```python
from build123d import *

# Parameters (mm, degrees)
SKETCH_R             = 10.3
PAD_DEPTH            = 2.9
SKETCH001_R          = 7.4
PAD001_DEPTH         = 19
SKETCH002_W          = 13.2
SKETCH002_H          = 4.5
POCKET_DEPTH         = 20
SKETCH003_W          = 8
SKETCH003_H          = 4.5
POCKET001_DEPTH      = 1.901
POCKET002_DEPTH      = 6
SKETCH005_R          = 1.5
POCKET003_DEPTH      = 15
POCKET004_DEPTH      = 20
POCKET004_DEPTH_BACK = -20
SKETCH007_W          = 2.3
SKETCH007_H          = 1.5
POCKET005_DEPTH      = 10.301


with BuildPart() as part:
    # Sketch → Pad (new body)
    with BuildSketch(Plane.XY):
        Circle(SKETCH_R)
    extrude(amount=PAD_DEPTH)

    # Sketch001 (on Face3 of Pad) → Pad001 (join)
    with BuildSketch(Plane.XY.offset(2.9)):
        Circle(SKETCH001_R)
    extrude(amount=PAD001_DEPTH)

    # Sketch002 (on Face5 of Pad001) → Pocket (cut)
    with BuildSketch(Plane.XY.offset(21.9)):
        Rectangle(SKETCH002_W, SKETCH002_H)
    extrude(amount=-POCKET_DEPTH, mode=Mode.SUBTRACT)

    # Sketch003 (on Face10 of Pocket) → Pocket001 (cut, through all)
    with BuildSketch(Plane.XY.offset(1.9)):
        Rectangle(SKETCH003_W, SKETCH003_H)
    extrude(amount=-POCKET001_DEPTH, mode=Mode.SUBTRACT)

    # Sketch004 (on Face9 of Pocket001) → Pocket002 (cut)
    with BuildSketch(Plane.XY.offset(21.9)):
        with BuildLine():
            ThreePointArc((-6, 0), (0, -6), (6, 0))
            Line((-6, 0), (6, 0))
        make_face()
    extrude(amount=-POCKET002_DEPTH, mode=Mode.SUBTRACT)

    # Sketch005 (on Face13 of Pocket002) → Pocket003 (cut)
    with BuildSketch(Plane.XY.offset(15.9)):
        with Locations((0, -4)):
            Circle(SKETCH005_R)
    extrude(amount=-POCKET003_DEPTH, mode=Mode.SUBTRACT)

    # Sketch006 → Pocket004 (cut, two sides)
    with BuildSketch(Plane.XZ) as pocket004_sk:
        with BuildLine():
            ThreePointArc((-2.25, 19.25), (-4, 17.5), (-2.25, 15.75))
            Line((-2.25, 15.75), (2.25, 15.75))
            ThreePointArc((2.25, 15.75), (4, 17.5), (2.25, 19.25))
            Line((-2.25, 19.25), (2.25, 19.25))
        make_face()
    extrude(amount=-POCKET004_DEPTH, mode=Mode.SUBTRACT)
    extrude(pocket004_sk.sketch, amount=-POCKET004_DEPTH_BACK, mode=Mode.SUBTRACT)

    # Sketch007 → Pocket005 (cut, through all)
    with BuildSketch(Plane.XZ):
        with Locations((0, 20)):
            Rectangle(SKETCH007_W, SKETCH007_H)
    extrude(amount=-POCKET005_DEPTH, mode=Mode.SUBTRACT)


solid = part.part
```
For this review, take the finished solid that the model builds, in its own axes (mm). A direction names the side the tool comes from. Coordinates: 2 decimals unless noted, no trailing zeros. Write each loop counter-clockwise with the first axis right and the second up, starting at its lowest first coordinate (ties: lowest second). Pieces come first, ordered by that corner, then holes. Notation, with made-up numbers: (8.25, 52) - (12.25, 52) arc R29 cw to (12.25, 89) - close; hole circle Ø1 at (35, 3.5). An arc over 180 degrees is marked (long way). Answer in a Markdown table with one row per item. Add a question column.
Q1. For probe 1 along Y at (x, z) = (0, 7); probe 2 along Z at (x, y) = (-1.25, -9.5); probe 3 along Z at (x, y) = (-0.75, -5.25), list the stretches that pass through material, from the lowest coordinate up.
Q2. Tool access review of faces 1 (the cylindrical face through (-4, 4.6, 17.5)), 2 (the flat face through (-4, 0, 1)), 3 (the flat face through (-6.6, 0, 12)): name each direction out of +Z, -Z, +X, -X, +Y, -Y from which nothing blocks a thin tool from reaching the whole face with its end or side.
Q3. We need section D-D, the plane x = -6. State the section outline as (y, z) points.
Q4. We need section B-B, the plane y = 0. State the section outline as (x, z) points, and give its area (3 significant figures).
Q5. We need section A-A, the plane x = 0. State the section outline as (y, z) points.
Q6. For P1, Ø3.5, axis at y = -1, z = 16.5, coming from the -X side; P2, Ø10, axis at x = -1, y = -0.5, coming from the -Z side; P3, Ø1.5, axis at x = 0, z = 7, coming from the -Y side; P4, Ø3, axis at x = 5, y = -0.5, coming from the +Z side, all flat-tipped, find the tip position at first contact; note any pin that passes through.
Q7. Draft analysis for pull direction Y (two halves, no side actions). For faces 4 (the cylindrical face through (0, -6, 20)), 5 (the cylindrical face through (4, 4.6, 17.5)), 6 (the cylindrical face through (-0.963, 7.337, 12.267)), state which applies: +Y half, -Y half, draft (parallel to the pull), parting line (faces both ways), or undercut.
Q8. We need section C-C, the plane z = 14. State the section outline as (x, y) points, and give its area (3 significant figures).
Answer list:
| question | item | result |
|---|---|---|
| 1 | probe 1 | y = -7.4 to -5.5, -2.5 to -2.25, 2.25 to 7.4 |
| 1 | probe 2 | z = 0 to 2.9 |
| 1 | probe 3 | z = 0 to 0.9 |
| 2 | face 1 | +Y, -Y |
| 2 | face 2 | +Z, -Z |
| 2 | face 3 | +Z |
| 3 | outline | (-8.37, 0) - (8.37, 0) - (8.37, 2.9) - (4.33, 2.9) - (4.33, 21.9) - (2.25, 21.9) - (2.25, 1.9) - (-2.25, 1.9) - (-2.25, 21.9) - (-4.33, 21.9) - (-4.33, 2.9) - (-8.37, 2.9) - close |
| 4 | outline | (-10.3, 0) - (-4, 0) - (-4, 1.9) - (-6.6, 1.9) - (-6.6, 21.9) - (-7.4, 21.9) - (-7.4, 2.9) - (-10.3, 2.9) - close; (4, 0) - (10.3, 0) - (10.3, 2.9) - (7.4, 2.9) - (7.4, 21.9) - (6.6, 21.9) - (6.6, 1.9) - (4, 1.9) - close |
| 4 | area | 61.7 mm2 |
| 5 | outline | (-10.3, 0) - (-2.25, 0) - (-2.25, 15.75) - (-2.5, 15.75) - (-2.5, 0.9) - (-5.5, 0.9) - (-5.5, 15.75) - (-7.4, 15.75) - (-7.4, 2.9) - (-10.3, 2.9) - close; (-7.4, 19.25) - (-6, 19.25) - (-6, 21.9) - (-7.4, 21.9) - close; (2.25, 0) - (10.3, 0) - (10.3, 2.9) - (7.4, 2.9) - (7.4, 15.75) - (2.25, 15.75) - close; (2.25, 20.75) - (7.4, 20.75) - (7.4, 21.9) - (2.25, 21.9) - close |
| 6 | P1 | stops at x = -7.4 |
| 6 | P2 | stops at z = 0 |
| 6 | P3 | stops at y = -7.4 |
| 6 | P4 | stops at z = 1.9 |
| 7 | face 4 | undercut |
| 7 | face 5 | draft |
| 7 | face 6 | parting line |
| 8 | outline | circle Ø14.8 at (0, 0); hole (-6.6, -2.25) - (6.6, -2.25) - (6.6, 2.25) - (-6.6, 2.25) - close; hole circle Ø3 at (0, -4) |
| 8 | area | 106 mm2 |
